from build123d import *

# Parameters (mm, degrees)
SKETCH1_W                                      = 50
SKETCH1_H                                      = 35
BOSS_EXTRUDE2_DEPTH                            = 5
SKETCH2_R                                      = 2
CUT_EXTRUDE1_DEPTH                             = 31.923292192
SKETCH3_R                                      = 9
CUT_EXTRUDE2_DEPTH                             = 1.5
SKETCH6_R                                      = 1.5113
CUT_EXTRUDE5_DEPTH                             = 4.8
SKETCH7_R                                      = 1.63195
CUT_EXTRUDE6_DEPTH                             = 31.923292192
SKETCH8_R                                      = 1.95
BOSS_EXTRUDE3_DEPTH                            = 2
FILLET1_R                                      = 15
SKETCH10_R                                     = 2.8575
CUT_EXTRUDE9_DEPTH                             = 3
CSK_FOR_4_FLAT_HEAD_MACHINE_SCREW1_D           = 2.9464
CSK_FOR_4_FLAT_HEAD_MACHINE_SCREW1_CSINK_D     = 5.715
CSK_FOR_4_FLAT_HEAD_MACHINE_SCREW1_CSINK_ANGLE = 82
SKETCH23_R                                     = 1.397
CUT_EXTRUDE13_DEPTH                            = 32.008063467
SKETCH24_R                                     = 2.794
CUT_EXTRUDE14_DEPTH                            = 2.75
CHAMFER1_SIZE                                  = 0.25
FILLET2_R                                      = 0.5
CHAMFER2_SIZE                                  = 0.25


with BuildPart() as part:
    # Sketch1 → Boss-Extrude2 (new body)
    with BuildSketch(Plane(origin=(0, 0, 0), x_dir=(1, 0, 0), z_dir=(0, 1, 0))):
        Rectangle(SKETCH1_W, SKETCH1_H)
    extrude(amount=-BOSS_EXTRUDE2_DEPTH)

    # Sketch2 → Cut-Extrude1 (cut, through all)
    with BuildSketch(Plane(origin=(0, 0, 0), x_dir=(1, 0, 0), z_dir=(0, 1, 0))):
        with Locations(Location((0, 0, 0), (0, 0, 270))):
            Circle(SKETCH2_R)
    extrude(amount=-CUT_EXTRUDE1_DEPTH, mode=Mode.SUBTRACT)

    # Sketch3 → Cut-Extrude2 (cut)
    with BuildSketch(Plane.XZ.offset(5)):
        with Locations(Location((0, 0, 0), (0, 0, 270))):
            Circle(SKETCH3_R)
    extrude(amount=-CUT_EXTRUDE2_DEPTH, mode=Mode.SUBTRACT)

    # Sketch6 → Cut-Extrude5 (cut)
    with BuildSketch(Plane(origin=(0, 0, 0), x_dir=(1, 0, 0), z_dir=(0, 1, 0))):
        with Locations(Location((-16, 9, 0), (0, 0, 270))):
            Circle(SKETCH6_R)
        with Locations(Location((16, 9, 0), (0, 0, 270))):
            Circle(SKETCH6_R)
    extrude(amount=-CUT_EXTRUDE5_DEPTH, mode=Mode.SUBTRACT)

    # Sketch7 → Cut-Extrude6 (cut, through all)
    with BuildSketch(Plane(origin=(0, 0, 0), x_dir=(1, 0, 0), z_dir=(0, 1, 0))):
        with Locations(Location((-16, 4, 0), (0, 0, 270))):
            Circle(SKETCH7_R)
        with Locations(Location((16, 4, 0), (0, 0, 270))):
            Circle(SKETCH7_R)
    extrude(amount=-CUT_EXTRUDE6_DEPTH, mode=Mode.SUBTRACT)

    # Sketch8 → Boss-Extrude3 (add)
    with BuildSketch(Plane.XZ.offset(3.5)):
        with Locations(Location((-6, 0, 0), (0, 0, 270))):
            Circle(SKETCH8_R)
    extrude(amount=BOSS_EXTRUDE3_DEPTH)

    # Fillet1
    fillet1_edges = [part.edges().sort_by_distance(p)[0] for p in [
        (25, -2.5, 17.5),
        (-25, -2.5, 17.5),
        (-25, -2.5, -17.5),
        (25, -2.5, -17.5),
    ]]
    fillet(fillet1_edges, radius=FILLET1_R)

    # Sketch10 → Cut-Extrude9 (cut)
    with BuildSketch(Plane.XZ.offset(5)):
        with Locations(Location((-16, -4, 0), (0, 0, 270))):
            Circle(SKETCH10_R)
        with Locations(Location((16, -4, 0), (0, 0, 270))):
            Circle(SKETCH10_R)
    extrude(amount=-CUT_EXTRUDE9_DEPTH, mode=Mode.SUBTRACT)

    # CSK for #4 Flat Head Machine Screw1 (through all)
    with Locations(Plane(origin=(4.242640687, 0, -4.242640687), x_dir=(0, 0, 1), z_dir=(0, 1, 0))):
        with Locations((0, 0), (8.485281374, 0), (8.485281374, -8.485281374), (0, -8.485281374)):
            CounterSinkHole(CSK_FOR_4_FLAT_HEAD_MACHINE_SCREW1_D / 2, CSK_FOR_4_FLAT_HEAD_MACHINE_SCREW1_CSINK_D / 2, counter_sink_angle=CSK_FOR_4_FLAT_HEAD_MACHINE_SCREW1_CSINK_ANGLE)

    # Sketch23 → Cut-Extrude13 (cut, through all)
    with BuildSketch(Plane(origin=(0, 0, 0), x_dir=(1, 0, 0), z_dir=(0, 1, 0))):
        with Locations(Location((-0.176776695, 6.894291117, 0), (0, 0, 270))):
            Circle(SKETCH23_R)
        with Locations(Location((6.894291117, -0.176776695, 0), (0, 0, 270))):
            Circle(SKETCH23_R)
    extrude(amount=-CUT_EXTRUDE13_DEPTH, mode=Mode.SUBTRACT)

    # Sketch24 → Cut-Extrude14 (cut)
    with BuildSketch(Plane.XZ.offset(5)):
        with Locations(Location((6.894291117, 0.176776695, 0), (0, 0, 270))):
            Circle(SKETCH24_R)
        with Locations(Location((-0.176776695, -6.894291117, 0), (0, 0, 270))):
            Circle(SKETCH24_R)
    extrude(amount=-CUT_EXTRUDE14_DEPTH, mode=Mode.SUBTRACT)

    # Chamfer1
    chamfer1_edges = [part.edges().sort_by_distance(p)[0] for p in [
        (-6, -5.5, 1.95),
    ]]
    chamfer(chamfer1_edges, length=CHAMFER1_SIZE)

    # Fillet2
    fillet2_edges = [part.edges().sort_by_distance(p)[0] for p in [
        (0, 0, -17.5),
        (0, -5, -17.5),
        (25, 0, 0),
        (-25, 0, 0),
        (0, 0, 17.5),
        (-20.606601718, 0, 13.106601718),
        (20.606601718, 0, 13.106601718),
        (20.606601718, 0, -13.106601718),
        (-20.606601718, 0, -13.106601718),
        (-25, -5, 0),
        (25, -5, 0),
        (0, -5, 17.5),
        (-20.606601718, -5, 13.106601718),
        (20.606601718, -5, 13.106601718),
        (20.606601718, -5, -13.106601718),
        (-20.606601718, -5, -13.106601718),
    ]]
    fillet(fillet2_edges, radius=FILLET2_R)

    # Chamfer2
    chamfer2_edges = [part.edges().sort_by_distance(p)[0] for p in [
        (-0.176776695, 0, -8.291291117),
        (6.894291117, 0, -1.220223305),
        (0, 0, -2),
        (-16, 0, -10.5113),
        (16, 0, -10.5113),
        (-16, 0, -5.63195),
        (16, 0, -5.63195),
    ]]
    chamfer(chamfer2_edges, length=CHAMFER2_SIZE)


solid = part.part
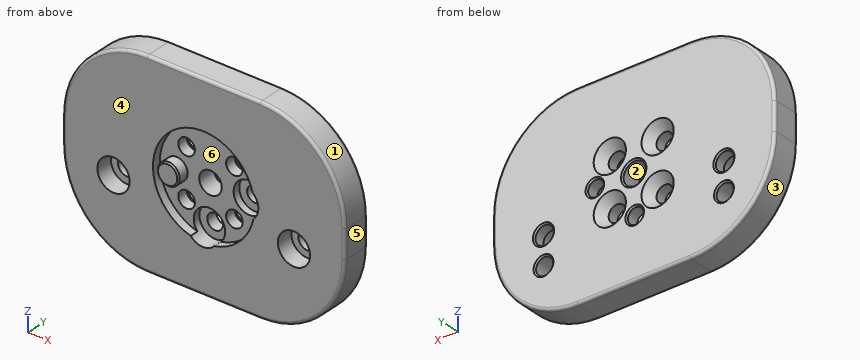
Input: part model. Units: mm. Frame: model coordinates. Face numbers are marked on the shaded views. A direction names the side the tool comes from. Give positions to 0.01 mm unless a question says otherwise; leave off trailing zeros. Write item = value, one per line. Start each with the question number.
1) Cut plane A-A on z = 0. Count the separate pieces of the cut face and the enclosed holes in it, then the cut area to 3 significant figures.
2) First-contact query: pin 1 Ø6.5 at (x, z) = (-0.18, -6.89) entering from -Y; pin 2 Ø1.7 at (x, z) = (16.5, -3) entering from -Y; pin 3 Ø1.7 at (x, z) = (8, -1) entering from -Y. Flat tips, straight axial feed; report the tip coordinate or a pass-through.
3) Draft query along X for the marked faces 1, 2, 3 and 4. Return one class per face: +X half, -X half, draft (parallel to the pull), parting line (faces both ways), or undercut.
4) Reachability of the marked faces 5 and 6 from +Z, -Z, +X, -X, +Y, -Y: full face, straight path, thin tool, end or side. Return the list, or none.
5) Material intervals for line 1 along X through (y, z) = (-3.9, 0); line 2 along Z through (x, y) = (0, -3.65); line 3 along Z through (x, y) = (4.5, -2.05), sorted ascending. Write a range as [from, to].
Solved:
q1.separate_pieces = 3
q1.enclosed_holes = 0
q1.area = 202 mm2
q2.pin_1 = -5
q2.pin_2 = -2
q2.pin_3 = -2.25
q3.face_1 = +X half
q3.face_2 = undercut
q3.face_3 = -X half
q3.face_4 = draft
q4.face_5 = +Z, -Z, +X, +Y, -Y
q4.face_6 = -Y
q5.line_1 = [-25, -9], [-7.95, -4.05], [9.68, 25]
q5.line_2 = [-17.5, -9.68], [9, 17.5]
q5.line_3 = [-17.5, -5.69], [-2.79, 2.79], [5.69, 17.5]
